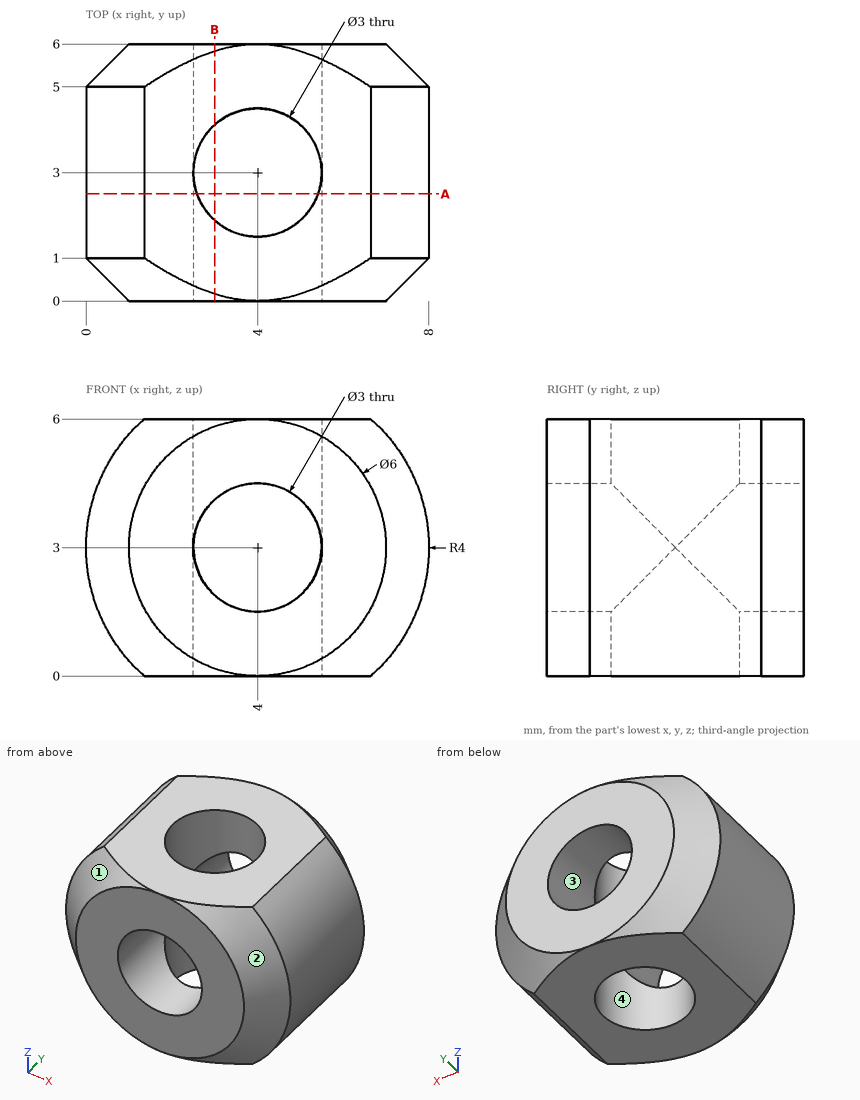
For this review, use the dimensioned drawing (mm, ordinates from the lowest corner) and the shaded views. Coordinates: 2 decimals unless noted, no trailing zeros. Order: outer loops, then holes, each group sorted by start corner. A loop starts at its lowest first (then second) coordinate and runs counter-clockwise, first axis right, second up. Notation, with made-up numbers: M 3.25,35.25 L 38.25,35.25 A15 cw 38.25,51.25 Z; hole C 63,-35 d5. An arc over 180 degrees is marked long. Answer as a JSON object with one key per item and string values. Group by question number.
1) For pin 1 (2.5 mm diameter, centred on x = 4, z = 3, fed in from +Y); pin 2 (1.5 mm diameter, centred on x = 5.5, z = 1, fed in from -Y); pin 3 (1 mm diameter, centred on y = 2, z = 1.5, fed in from +X), all flat-tipped, find the tip position at first contact; note any pin that passes through.
2) Wall thickness on L1, parallel to Y at x = 4, z = 4.7; L2, parallel to X at y = 1.7, z = 3; L3, parallel to X at y = 4.95, z = 2.5: over which ranges is each line inside the solid? List them lowest first.
3) Add section A-A, the plane y = 2.5. Write out the cut boundary in (x, z).
4) Add section B-B, the plane x = 3. Count the separate pieces of the cut face and the enclosed holes in it, then the cut area to 3 significant figures.
5) Mouldability with a two-part tool opening along X and no side actions: class the marked faces 1, 2, 3 and 4 as pulls with the +X half, pulls with the -X half, needs draft (parallel to the pull), parting line crosses it, or undercut.
Computed values:
{
 "1": {"pin 1": "passes through", "pin 2": "stops at y = 0", "pin 3": "stops at x = 7.87"},
 "2": {"L1": "y = 0 to 1.5, 4.5 to 6", "L2": "x = 0 to 2.5, 5.5 to 8", "L3": "x = 0.03 to 2.59, 5.41 to 7.97"},
 "3": {"outline": "M 1.35,0 L 2.59,0 L 2.59,2.5 A1.5 cw 2.59,3.5 L 2.59,6 L 1.35,6 A4 ccw Z; M 5.41,0 L 6.65,0 A4 ccw 6.65,6 L 5.41,6 L 5.41,3.5 A1.5 cw 5.41,2.5 Z"},
 "4": {"separate pieces": "4", "enclosed holes": "0", "area": "14.1 mm^2"},
 "5": {"face 1": "pulls with the -X half", "face 2": "pulls with the +X half", "face 3": "undercut", "face 4": "undercut"}
}
